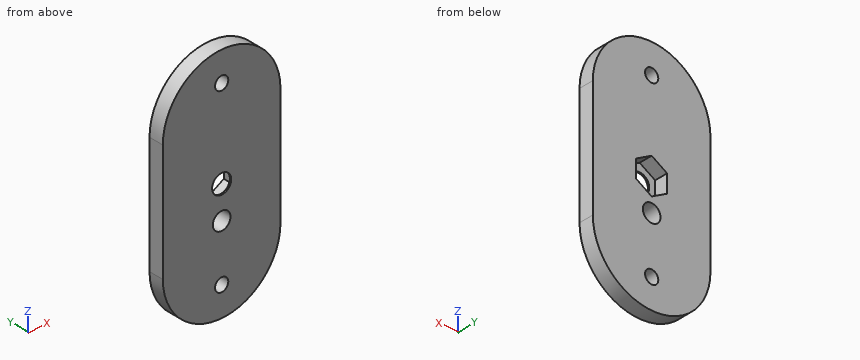
Autodesk Inventor part; units mm, degrees
ref_plane "YZ Plane" through (0, 0, 0) normal (1, 0, 0) x (0, 1, 0)
ref_plane "XZ Plane" through (0, 0, 0) normal (0, 1, 0) x (-1, 0, 0)
ref_plane "XY Plane" through (0, 0, 0) normal (0, 0, 1) x (1, 0, 0)
sketch "Sketch1" plane through (0, 0, 0) normal (0, 1, 0) x (-1, 0, 0)
  line L0 (0, 40) -> (0, 40)
  line L1 (-20, 20) -> (-20, -20)
  line L2 (0, -40) -> (0, -40)
  line L3 (20, -20) -> (20, 20)
  line L4 (20, 40) -> (-20, -40) construction
  line L5 (-20, 40) -> (20, -40) construction
  arc A0 (0, -40) -> (20, -20) centre (0, -20) ccw
  arc A1 (20, 20) -> (0, 40) centre (0, 20) ccw
  arc A2 (0, 40) -> (-20, 20) centre (0, 20) ccw
  arc A3 (-20, -20) -> (0, -40) centre (0, -20) ccw
  point P0 (0, 0)
  dimension "d0" = 40
  dimension "d1" = 80
  dimension "d18" = 20
extrude "Extrusion1" add sketch "Sketch1" along normal blind 5
sketch "Sketch2" plane through (0, 5, 0) normal (0, 1, 0) x (1, 0, 0)
  line L0 (-5.25, 3.0311) -> (0, 6.0622)
  line L1 (0, 6.0622) -> (5.25, 3.0311)
  line L2 (5.25, 3.0311) -> (5.25, -3.0311)
  line L3 (5.25, -3.0311) -> (0, -6.0622)
  line L4 (0, -6.0622) -> (-5.25, -3.0311)
  line L5 (-5.25, -3.0311) -> (-5.25, 3.0311)
  point P0 (0, 0)
  point P1 (0, 0)
  point P2 (5.25, 0)
  point P3 (-5.25, 0)
  dimension "d4" = 10.5
extrude "Extrusion2" cut sketch "Sketch2" against normal blind 4.5
sketch "Sketch3" plane through (0, 0.5, 0) normal (0, 1, 0) x (1, 0, 0)
  circle A0 centre (0, 0) radius 3.25
  dimension "d7" = 6.5
extrude "Extrusion3" cut sketch "Sketch3" against normal through all
sketch "Sketch4" plane through (0, 0, 0) normal (0, -1, 0) x (1, 0, 0)
  circle A0 centre (0, -11) radius 3
  circle A1 centre (0, 30) radius 2.25
  circle A2 centre (0, -30) radius 2.25
  point P0 (0, 0)
  dimension "d10" = 6
  dimension "d11" = 11
  dimension "d12" = 4.5
  dimension "d13" = 4.5
  dimension "d14" = 30
  dimension "d15" = 30
extrude "Extrusion4" cut sketch "Sketch4" against normal through all
properties part number "Tripod mount"
Build history of the part. All positions in model axes, mm. Coordinates: 2 decimals unless noted, no trailing zeros. Write each loop counter-clockwise with the first axis right and the second up, starting at its lowest first coordinate (ties: lowest second). Pieces come first, ordered by that corner, then holes. Notation, with made-up numbers: (64.25, -33.75) -> (118.25, -33.75) arc R31 cw to (118.25, 1.25) -> close; hole circle Ø5 at (83, 86). An arc over 180 degrees is marked (long way). Use CSV: the item, a comma, the result in double quotes. Start each with the question number.
Q1. Cut at D-D, the plane x = 9. List the corners of the cut face in (y, z), then the cut area to 3 significant figures.
Q2. Flat gauge pin, fed straight in: pin 1 Ø4 at (x, z) = (0, 0) entering from +Y. Where does the tip first touch, or does it go through?
Q3. Cut at C-C, the plane z = 30. List the corners of the cut face in (x, y).
Q4. Cut at A-A, the plane z = -11. List the corners of the cut face in (x, y), then the cut area to 3 significant figures.
Q5. Cut at B-B, the plane y = 3.5. List the corners of the cut face in (x, z).
Q6. Drill centre lines: probe 1 along Z at (x, y) = (0, 3.8); probe 2 along Z at (x, y) = (0, 0.35); probe 3 along X at (y, z) = (0.4, 0). Where is each one in solid material? Low to high.
Checked values:
1,outline,"(0, -37.86) -> (5, -37.86) -> (5, 37.86) -> (0, 37.86) -> close"
1,area,"379 mm²"
2,pin 1,"passes through"
3,outline,"(-17.32, 0) -> (-2.25, 0) -> (-2.25, 5) -> (-17.32, 5) -> close; (2.25, 0) -> (17.32, 0) -> (17.32, 5) -> (2.25, 5) -> close"
4,outline,"(-20, 0) -> (-3, 0) -> (-3, 5) -> (-20, 5) -> close; (3, 0) -> (20, 0) -> (20, 5) -> (3, 5) -> close"
4,area,"170 mm²"
5,outline,"(-20, -20) arc R20 ccw to (20, -20) -> (20, 20) arc R20 ccw to (-20, 20) -> close; hole (-5.25, -3.03) -> (0, -6.06) -> (5.25, -3.03) -> (5.25, 3.03) -> (0, 6.06) -> (-5.25, 3.03) -> close; hole circle Ø6 at (0, -11); hole circle Ø4.5 at (0, -30); hole circle Ø4.5 at (0, 30)"
6,probe 1,"z = -40 to -32.25, -27.75 to -14, -8 to -6.06, 6.06 to 27.75, 32.25 to 40"
6,probe 2,"z = -40 to -32.25, -27.75 to -14, -8 to -3.25, 3.25 to 27.75, 32.25 to 40"
6,probe 3,"x = -20 to -3.25, 3.25 to 20"
